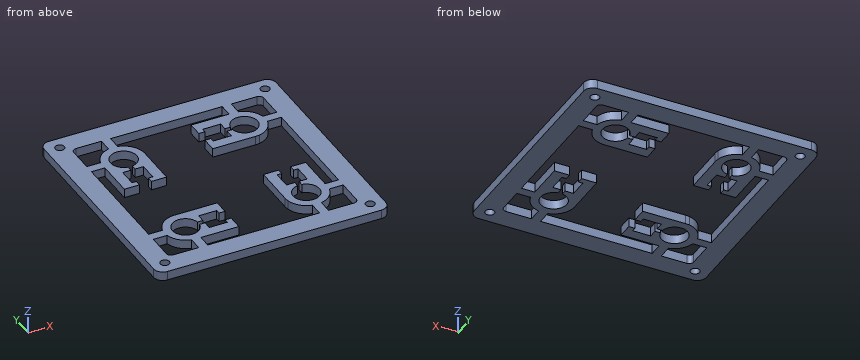
```python
from build123d import *

# Parameters (mm, degrees)
SKETCH_1_R               = 1.5
SKETCH_1_R_2             = 4.35
EXTRUDE_1_DEPTH          = 3
EXTRUDE_3_DEPTH          = 3
CUT_EXTRUDE_2_DEPTH      = 55.459204915
PATTERN_CIRCULAR_2_COUNT = 4


with BuildPart() as part:
    # Sketch 1 → Extrude 1 (new body)
    with BuildSketch(Plane.XY):
        with BuildLine():
            Line((-35.45, 38.45), (35.45, 38.45))
            ThreePointArc((35.45, 38.45), (37.571320344, 37.571320344), (38.45, 35.45))
            Line((38.45, 35.45), (38.45, -35.45))
            ThreePointArc((38.45, -35.45), (37.571320344, -37.571320344), (35.45, -38.45))
            Line((35.45, -38.45), (-35.45, -38.45))
            ThreePointArc((-35.45, -38.45), (-37.571320344, -37.571320344), (-38.45, -35.45))
            Line((-38.45, -35.45), (-38.45, 35.45))
            ThreePointArc((-38.45, 35.45), (-37.571320344, 37.571320344), (-35.45, 38.45))
        make_face()
        with Locations((-34, 34)):
            Circle(SKETCH_1_R, mode=Mode.SUBTRACT)
        with Locations((34, 34)):
            Circle(SKETCH_1_R, mode=Mode.SUBTRACT)
        with Locations((34, -34)):
            Circle(SKETCH_1_R, mode=Mode.SUBTRACT)
        with Locations((-34, -34)):
            Circle(SKETCH_1_R, mode=Mode.SUBTRACT)
        with Locations((-20, 20)):
            Circle(SKETCH_1_R_2, mode=Mode.SUBTRACT)
        with Locations((20, 20)):
            Circle(SKETCH_1_R_2, mode=Mode.SUBTRACT)
        with Locations((-20, -20)):
            Circle(SKETCH_1_R_2, mode=Mode.SUBTRACT)
        with Locations((20, -20)):
            Circle(SKETCH_1_R_2, mode=Mode.SUBTRACT)
        with BuildLine():
            Line((-29.95, -31.45), (-21.5, -31.45))
            Line((-21.5, -31.45), (-21.5, -26.837397166))
            ThreePointArc((-21.5, -26.837397166), (-24.949747468, -24.949747468), (-26.837397166, -21.5))
            Line((-26.837397166, -21.5), (-31.45, -21.5))
            Line((-31.45, -21.5), (-31.45, -29.95))
            ThreePointArc((-31.45, -29.95), (-31.010660172, -31.010660172), (-29.95, -31.45))
        make_face(mode=Mode.SUBTRACT)
        with BuildLine():
            Line((31.45, 29.95), (31.45, 21.5))
            Line((31.45, 21.5), (26.837397166, 21.5))
            ThreePointArc((26.837397166, 21.5), (24.949747468, 24.949747468), (21.5, 26.837397166))
            Line((21.5, 26.837397166), (21.5, 31.45))
            Line((21.5, 31.45), (29.95, 31.45))
            ThreePointArc((29.95, 31.45), (31.010660172, 31.010660172), (31.45, 29.95))
        make_face(mode=Mode.SUBTRACT)
        with BuildLine():
            Line((-29.95, 31.45), (-21.5, 31.45))
            Line((-21.5, 31.45), (-21.5, 26.837397166))
            ThreePointArc((-21.5, 26.837397166), (-24.949747468, 24.949747468), (-26.837397166, 21.5))
            Line((-26.837397166, 21.5), (-31.45, 21.5))
            Line((-31.45, 21.5), (-31.45, 29.95))
            ThreePointArc((-31.45, 29.95), (-31.010660172, 31.010660172), (-29.95, 31.45))
        make_face(mode=Mode.SUBTRACT)
        with BuildLine():
            Line((-18.5, 31.45), (18.5, 31.45))
            Line((18.5, 31.45), (18.5, 26.837397166))
            ThreePointArc((18.5, 26.837397166), (15.050252532, 24.949747468), (13.162602834, 21.5))
            Line((13.162602834, 21.5), (-13.162602834, 21.5))
            ThreePointArc((-13.162602834, 21.5), (-15.050252532, 24.949747468), (-18.5, 26.837397166))
            Line((-18.5, 26.837397166), (-18.5, 31.45))
        make_face(mode=Mode.SUBTRACT)
        with BuildLine():
            Line((-31.45, 18.5), (-31.45, -18.5))
            Line((-31.45, -18.5), (-26.837397166, -18.5))
            ThreePointArc((-26.837397166, -18.5), (-24.949747468, -15.050252532), (-21.5, -13.162602834))
            Line((-21.5, -13.162602834), (-21.5, 13.162602834))
            ThreePointArc((-21.5, 13.162602834), (-24.949747468, 15.050252532), (-26.837397166, 18.5))
            Line((-26.837397166, 18.5), (-31.45, 18.5))
        make_face(mode=Mode.SUBTRACT)
        with BuildLine():
            Line((-13.162602834, 18.5), (13.162602834, 18.5))
            ThreePointArc((13.162602834, 18.5), (15.050252532, 15.050252532), (18.5, 13.162602834))
            Line((18.5, 13.162602834), (18.5, -13.162602834))
            ThreePointArc((18.5, -13.162602834), (15.050252532, -15.050252532), (13.162602834, -18.5))
            Line((13.162602834, -18.5), (-13.162602834, -18.5))
            ThreePointArc((-13.162602834, -18.5), (-15.050252532, -15.050252532), (-18.5, -13.162602834))
            Line((-18.5, -13.162602834), (-18.5, 13.162602834))
            ThreePointArc((-18.5, 13.162602834), (-15.050252532, 15.050252532), (-13.162602834, 18.5))
        make_face(mode=Mode.SUBTRACT)
        with BuildLine():
            Line((26.837397166, 18.5), (31.45, 18.5))
            Line((31.45, 18.5), (31.45, -18.5))
            Line((31.45, -18.5), (26.837397166, -18.5))
            ThreePointArc((26.837397166, -18.5), (24.949747468, -15.050252532), (21.5, -13.162602834))
            Line((21.5, -13.162602834), (21.5, 13.162602834))
            ThreePointArc((21.5, 13.162602834), (24.949747468, 15.050252532), (26.837397166, 18.5))
        make_face(mode=Mode.SUBTRACT)
        with BuildLine():
            Line((-18.5, -31.45), (-18.5, -26.837397166))
            ThreePointArc((-18.5, -26.837397166), (-15.050252532, -24.949747468), (-13.162602834, -21.5))
            Line((-13.162602834, -21.5), (13.162602834, -21.5))
            ThreePointArc((13.162602834, -21.5), (15.050252532, -24.949747468), (18.5, -26.837397166))
            Line((18.5, -26.837397166), (18.5, -31.45))
            Line((18.5, -31.45), (-18.5, -31.45))
        make_face(mode=Mode.SUBTRACT)
        with BuildLine():
            Line((21.5, -26.837397166), (21.5, -31.45))
            Line((21.5, -31.45), (29.95, -31.45))
            ThreePointArc((29.95, -31.45), (31.010660172, -31.010660172), (31.45, -29.95))
            Line((31.45, -29.95), (31.45, -21.5))
            Line((31.45, -21.5), (26.837397166, -21.5))
            ThreePointArc((26.837397166, -21.5), (24.949747468, -24.949747468), (21.5, -26.837397166))
        make_face(mode=Mode.SUBTRACT)
    extrude(amount=EXTRUDE_1_DEPTH)

    # Sketch 2 → Extrude 3 (add)
    with BuildSketch(Plane(origin=(0, 0, 0), x_dir=(-1, 0, 0), z_dir=(0, 0, -1))):
        with BuildLine():
            ThreePointArc((16.55, 13.909228292), (13.952273154, 16.475088654), (13, 20))
            Line((13, 20), (13, 5.9))
            Line((13, 5.9), (15.009228292, 3.9))
            Line((15.009228292, 3.9), (24.990771708, 3.9))
            Line((24.990771708, 3.9), (27, 5.9))
            Line((27, 5.9), (27, 20))
            ThreePointArc((27, 20), (26.047726846, 16.475088654), (23.45, 13.909228292))
            Line((23.45, 13.909228292), (23.45, 7.9))
            Line((23.45, 7.9), (16.55, 7.9))
            Line((16.55, 7.9), (16.55, 13.909228292))
        make_face()
    extrude_3 = extrude(amount=-EXTRUDE_3_DEPTH)

    # Sketch 4 → Cut-Extrude 2 (cut, through all)
    with BuildSketch(Plane(origin=(0, 0, 0), x_dir=(-1, 0, 0), z_dir=(0, 0, -1))):
        with BuildLine():
            Line((16.55, 7.9), (16.55, 7.899228292))
            Line((16.55, 7.899228292), (18, 7.899228292))
            Line((18, 7.899228292), (18, 5.9))
            Line((18, 5.9), (13, 5.9))
            Line((13, 5.9), (15.009228292, 3.9))
            Line((15.009228292, 3.9), (18.5, 3.9))
            Line((18.5, 3.9), (18.5, -13))
            Line((18.5, -13), (20, -13))
            ThreePointArc((20, -13), (20.754393744, -13.040769433), (21.5, -13.162602834))
            Line((21.5, -13.162602834), (21.5, 3.9))
            Line((21.5, 3.9), (24.990771708, 3.9))
            Line((24.990771708, 3.9), (27, 5.9))
            Line((27, 5.9), (22, 5.9))
            Line((22, 5.9), (22, 7.899228292))
            Line((22, 7.899228292), (23.45, 7.899228292))
            Line((23.45, 7.899228292), (23.45, 7.9))
            Line((23.45, 7.9), (21.5, 7.9))
            Line((21.5, 7.9), (21.5, 13.162602834))
            ThreePointArc((21.5, 13.162602834), (22.502995684, 13.4627978), (23.45, 13.909228292))
            Line((23.45, 13.909228292), (20.7, 13.909228292))
            Line((20.7, 13.909228292), (20.7, 15.706691253))
            ThreePointArc((20.7, 15.706691253), (20, 15.65), (19.3, 15.706691253))
            Line((19.3, 15.706691253), (19.3, 13.909228292))
            Line((19.3, 13.909228292), (16.55, 13.909228292))
            ThreePointArc((16.55, 13.909228292), (17.497004316, 13.4627978), (18.5, 13.162602834))
            Line((18.5, 13.162602834), (18.5, 7.9))
            Line((18.5, 7.9), (16.55, 7.9))
        make_face()
    cut_extrude_2 = extrude(amount=-CUT_EXTRUDE_2_DEPTH, mode=Mode.SUBTRACT)

    # Pattern Circular 2: Extrude 3, Cut-Extrude 2 ×4 about axis
    pattern_circular_2_axis = Axis((0, 0, 0), (0, 0, 1))
    add([extrude_3.rotate(pattern_circular_2_axis, i * 360 / PATTERN_CIRCULAR_2_COUNT) for i in range(1, PATTERN_CIRCULAR_2_COUNT)])
    add([cut_extrude_2.rotate(pattern_circular_2_axis, i * 360 / PATTERN_CIRCULAR_2_COUNT) for i in range(1, PATTERN_CIRCULAR_2_COUNT)], mode=Mode.SUBTRACT)


solid = part.part
```
The model under review builds one solid part; all positions refer to its coordinate system, in mm. Coordinates: 2 decimals unless noted, no trailing zeros. Write each loop counter-clockwise with the first axis right and the second up, starting at its lowest first coordinate (ties: lowest second). Pieces come first, ordered by that corner, then holes. Notation, with made-up numbers: (77.5, -4) - (85.5, -4) arc R31 cw to (85.5, 23) - close; hole circle Ø11 at (77, -9.75). An arc over 180 degrees is marked (long way). Answer in a Markdown table with one row per item. Add a question column.
Q1. Consider section B-B on y = -34. Give the boundary of the cut face in (x, z), then the cut area to 3 significant figures.
Q2. To check wall thickness, follow line 1 along X through (y, z) = (-8, 2.15); line 2 along X through (y, z) = (-20, 1). State the ranges of each line that lie inside material, in increasing order. Write a range as from..to.
Q3. Clearance check with a flat-ended pin moving along its axis: pin 1 (10 mm diameter, centred on x = -20, y = -20, fed in from -Z). State where the tip first meets the part, or that it passes through.
Q4. Consider section D-D on y = -12. Give the boundary of the cut face in (x, z).
Q5. Consider section A-A on x = 3. Give the boundary of the cut face in (y, z), then the cut area to 3 significant figures.
Answers below:
| question | item | result |
|---|---|---|
| 1 | outline | (-38.45, 0) - (-35.5, 0) - (-35.5, 3) - (-38.45, 3) - close; (-32.5, 0) - (32.5, 0) - (32.5, 3) - (-32.5, 3) - close; (35.5, 0) - (38.45, 0) - (38.45, 3) - (35.5, 3) - close |
| 1 | area | 213 mm² |
| 2 | line 1 | -38.45..-31.45, 13..16.55, 23.45..27, 31.45..38.45 |
| 2 | line 2 | -38.45..-24.35, 13..15.65, 24.35..38.45 |
| 3 | pin 1 | z = 0 |
| 4 | outline | (-38.45, 0) - (-31.45, 0) - (-31.45, 3) - (-38.45, 3) - close; (13, 0) - (16.55, 0) - (16.55, 3) - (13, 3) - close; (23.45, 0) - (27, 0) - (27, 3) - (23.45, 3) - close; (31.45, 0) - (38.45, 0) - (38.45, 3) - (31.45, 3) - close |
| 5 | outline | (-38.45, 0) - (-31.45, 0) - (-31.45, 3) - (-38.45, 3) - close; (31.45, 0) - (38.45, 0) - (38.45, 3) - (31.45, 3) - close |
| 5 | area | 42.0 mm² |
